Job drawing, mm, ordinate dimensions from the low corner. One solid piece. Give positions to 0.01 mm unless a question says otherwise; leave off trailing zeros. Order: outer loops, then holes, each group sorted by start corner. A loop starts at its lowest first (then second) coordinate and runs counter-clockwise, first axis right, second up.
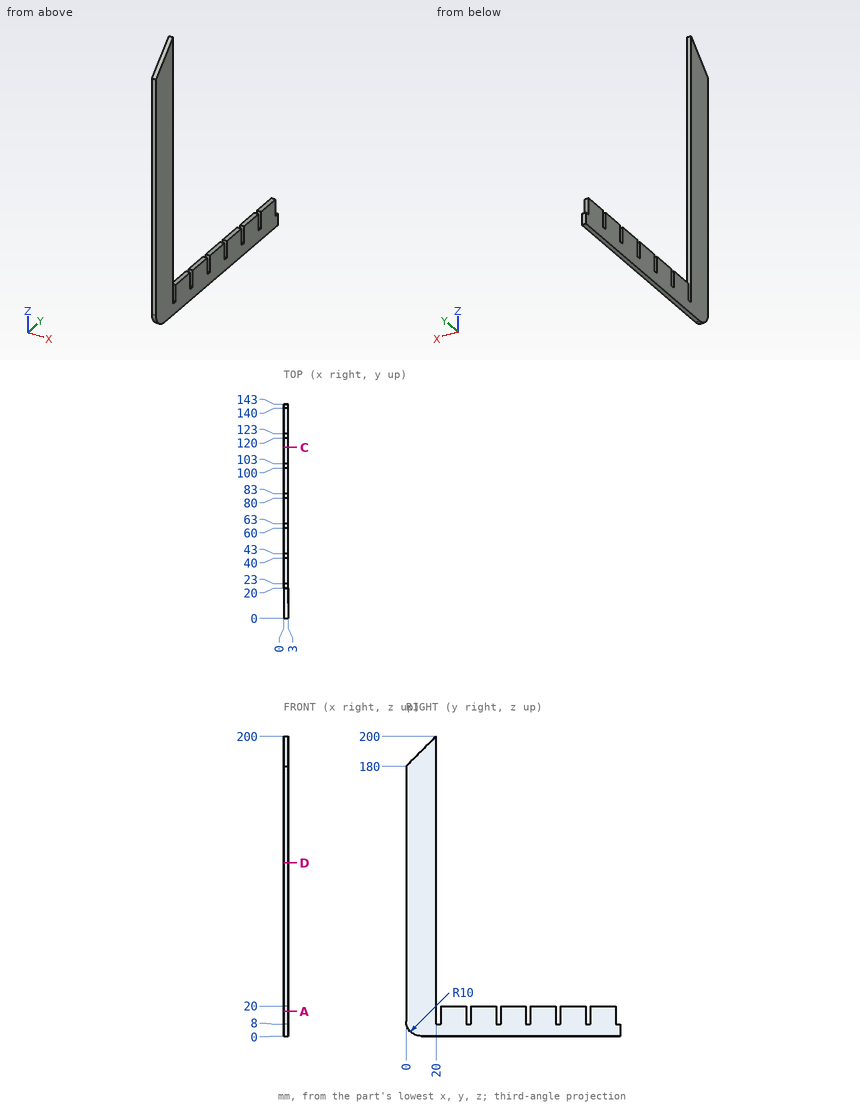
Item 1: Drill centre lines: probe 1 along Y at (x, z) = (2.9, 26); probe 2 along Z at (x, y) = (2.4, 102.5). Where is each one in solid material? Low to high.
Item 2: Band-saw the part on C-C on y = 114. List the corners of the cut face in (x, z).
Item 3: Drop flat-ended pins along their axis: P1, Ø1.5, axis at x = 1, y = 57.5, coming from the -Z side; P2, Ø1.5, axis at x = 1.5, y = 42, coming from the +Z side; P3, Ø6, axis at y = 51, z = 24, coming from the -X side; P4, Ø0.9, axis at x = 2, z = 16.5, coming from the +Y side. Give the stop position or say it passes through.
Item 4: Band-saw the part on A-A on z = 16.5. List the corners of the cut face in (x, y).
Working result:
1. probe 1: y = 0 to 20
1. probe 2: z = 0 to 8
2. outline: (0, 0) - (3, 0) - (3, 20) - (0, 20) - close
3. P1: stops at z = 0
3. P2: stops at z = 8
3. P3: passes through
3. P4: stops at y = 140
4. outline: (0, 0) - (3, 0) - (3, 20) - (0, 20) - close; (0, 23) - (3, 23) - (3, 40) - (0, 40) - close; (0, 43) - (3, 43) - (3, 60) - (0, 60) - close; (0, 63) - (3, 63) - (3, 80) - (0, 80) - close; (0, 83) - (3, 83) - (3, 100) - (0, 100) - close; (0, 103) - (3, 103) - (3, 120) - (0, 120) - close; (0, 123) - (3, 123) - (3, 140) - (0, 140) - close
